For this review, use the dimensioned drawing (mm, ordinates from the lowest corner) and the shaded views. Give positions to 0.01 mm unless a question says otherwise; leave off trailing zeros. Loops run counter-clockwise (first coordinate to the right, second up) from the corner with the lowest first, then second, coordinate; pieces in that order, holes last. Notation, with made-up numbers: M -36.5,34 L -32.5,34 A31 ccw -32.5,70 Z; hole C 5.25,1 d4. An arc over 180 degrees is marked long. Use CSV: the item, a comma, the result in double quotes. Start each with the question number.
1. The part is to be moulded in two halves that separate along X. For the marked faces 1, 2 and 3, say which applies: pulls with the +X half, pulls with the -X half, needs draft (parallel to the pull), parting line crosses it, or undercut.
2. Take a section at B-B, the plane y = 13.65. Write out the cut boundary in (x, z) (1 decimal).
3. To check wall thickness, follow line 1 (Y direction, x = 2.1, z = 0.5); line 2 (Y direction, x = 2.55, z = 0.8) (1 decimal); line 3 (Y direction, x = 3, z = 0.55) (1 decimal). State the ranges of each line that lie inside material, in increasing order. Write a range as [from, to].
4. Take a section at A-A, the plane x = 2.1. State how many separate pieces and enclosed holes the cut face has.
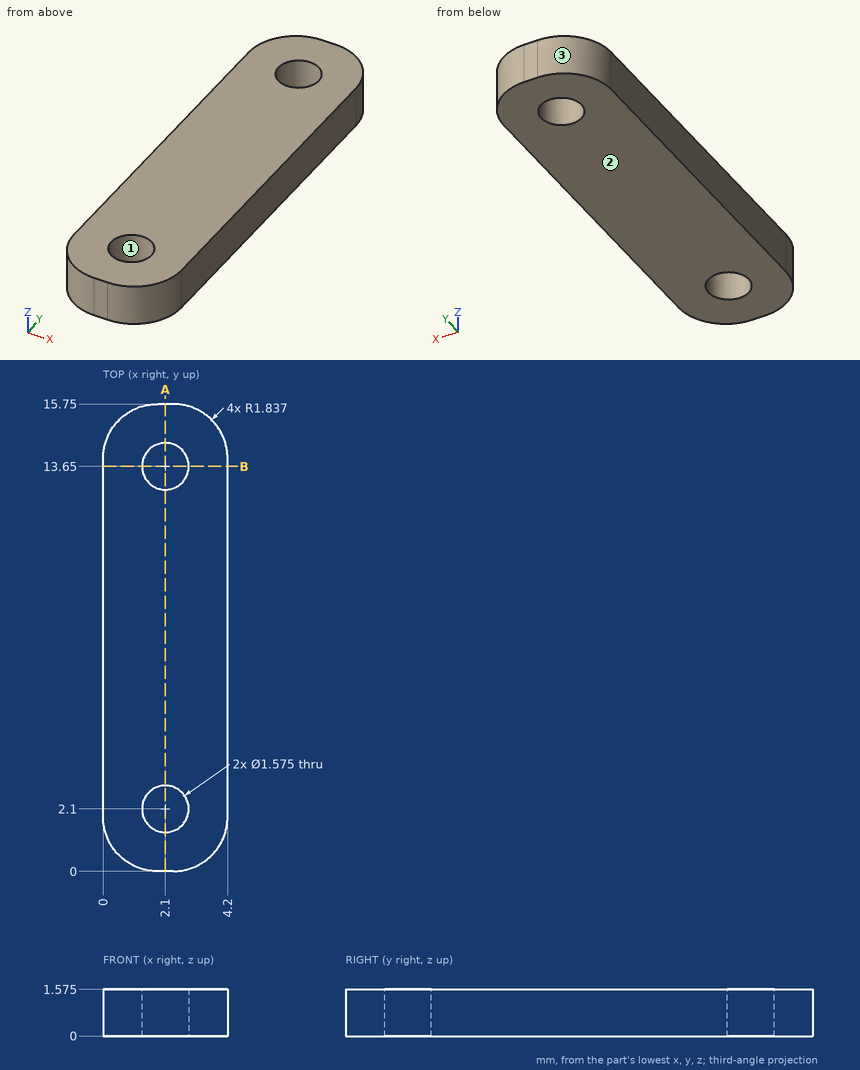
Result set:
1,face 1,"undercut"
1,face 2,"needs draft"
1,face 3,"pulls with the -X half"
2,outline,"M 0,0 L 1.3,0 L 1.3,1.6 L 0,1.6 Z; M 2.9,0 L 4.2,0 L 4.2,1.6 L 2.9,1.6 Z"
3,line 1,"[0, 1.31], [2.89, 12.86], [14.44, 15.75]"
3,line 2,"[0, 1.5], [2.7, 13], [14.3, 15.7]"
3,line 3,"[0.1, 15.6]"
4,separate pieces,"3"
4,enclosed holes,"0"
